Study the drawing (mm; zero at the part's minimum x, y, z) and answer. A direction names the side the tool comes from. Give positions to 0.01 mm unless a question says otherwise; leave off trailing zeros. Order: outer loops, then holes, each group sorted by start corner. A loop starts at its lowest first (then second) coordinate and runs counter-clockwise, first axis right, second up. Notation, with made-up numbers: (39.25, -23.5) - (45.25, -23.5) arc R8 ccw to (45.25, -19.5) - close; hole circle Ø6 at (30.5, -1). An arc over 180 degrees is marked (long way). Put each result on its own line as item: value.
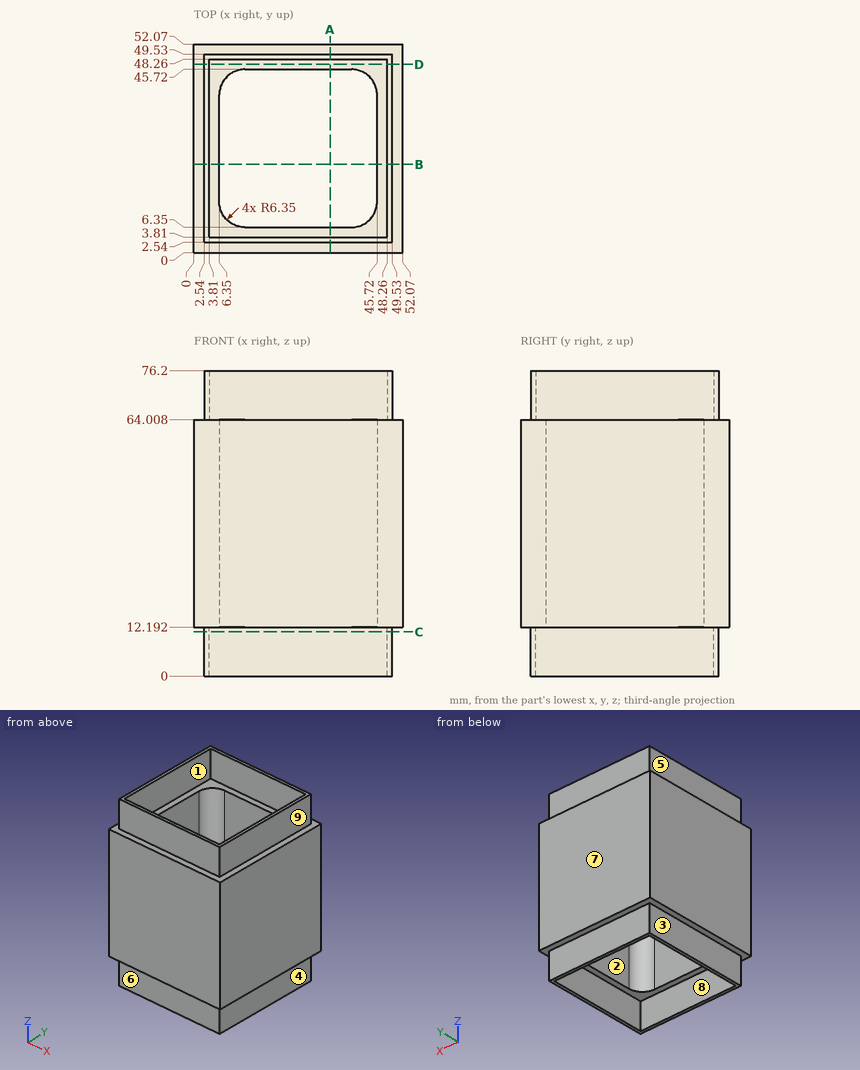
(1) Given pin 1 (6 mm diameter, centred on x = 23.5, z = 71.5, fed in from -Y); pin 2 (10 mm diameter, centred on x = 22.5, z = 72, fed in from +Y); pin 3 (3.5 mm diameter, centred on y = 15.5, z = 4, fed in from +X); pin 4 (2 mm diameter, centred on x = 9, y = 17.5, fed in from -Z), each flat-ended and moving along its own axis, determine where each tip first touches the part or whether it passes through.
Geometry check:
pin 1: stops at y = 2.54
pin 2: stops at y = 49.53
pin 3: stops at x = 49.53
pin 4: passes through
(2) Determine the mould class of the marked faces 6, 7, 8 and 9 for opening direction Y: pulls with the +Y half, pulls with the -Y half, needs draft (parallel to the pull), parting line crosses it, or undercut.
Geometry check:
face 6: pulls with the -Y half
face 7: pulls with the +Y half
face 8: undercut
face 9: needs draft
(3) Section C-C, the plane z = 11 is taken. Write down the section's boundary in (x, y).
Geometry check:
outline: (2.54, 2.54) - (49.53, 2.54) - (49.53, 49.53) - (2.54, 49.53) - close; hole (3.81, 3.81) - (48.26, 3.81) - (48.26, 48.26) - (3.81, 48.26) - close
(4) Section A-A, the plane x = 34 is taken. Write down the section's boundary in (y, z), then the cut area to 3 significant figures.
Geometry check:
outline: (0, 12.19) - (2.54, 12.19) - (2.54, 0) - (3.81, 0) - (3.81, 12.19) - (6.35, 12.19) - (6.35, 64.01) - (3.81, 64.01) - (3.81, 76.2) - (2.54, 76.2) - (2.54, 64.01) - (0, 64.01) - close; (45.72, 12.19) - (48.26, 12.19) - (48.26, 0) - (49.53, 0) - (49.53, 12.19) - (52.07, 12.19) - (52.07, 64.01) - (49.53, 64.01) - (49.53, 76.2) - (48.26, 76.2) - (48.26, 64.01) - (45.72, 64.01) - close
area: 720 mm²
(5) Section D-D, the plane y = 47 is taken. Write down the section's boundary in (x, z).
Geometry check:
outline: (0, 12.19) - (2.54, 12.19) - (2.54, 0) - (3.81, 0) - (3.81, 12.19) - (48.26, 12.19) - (48.26, 0) - (49.53, 0) - (49.53, 12.19) - (52.07, 12.19) - (52.07, 64.01) - (49.53, 64.01) - (49.53, 76.2) - (48.26, 76.2) - (48.26, 64.01) - (3.81, 64.01) - (3.81, 76.2) - (2.54, 76.2) - (2.54, 64.01) - (0, 64.01) - close
(6) Straight lines are drawn through the part: line 1 (Y direction, x = 38, z = 60.5); line 2 (X direction, y = 42, z = 72). For each, find the intervals that lie inside material, in ascending order.
Geometry check:
line 1: y = 0 to 6.35, 45.72 to 52.07
line 2: x = 2.54 to 3.81, 48.26 to 49.53
(7) A tool of negligible diameter and unlimited length cuts with its end or side. For the marked faces 1, 2, 3, 4 and 5, from which of +Z, -Z, +X, -X, +Y, -Y can it reach the whole face along a straight path? Write none if from no direction.
Geometry check:
face 1: +Z
face 2: +Z, -Z
face 3: -Z, -X, +Y, -Y
face 4: -Z, +X, +Y, -Y
face 5: +Z, -X, +Y, -Y
